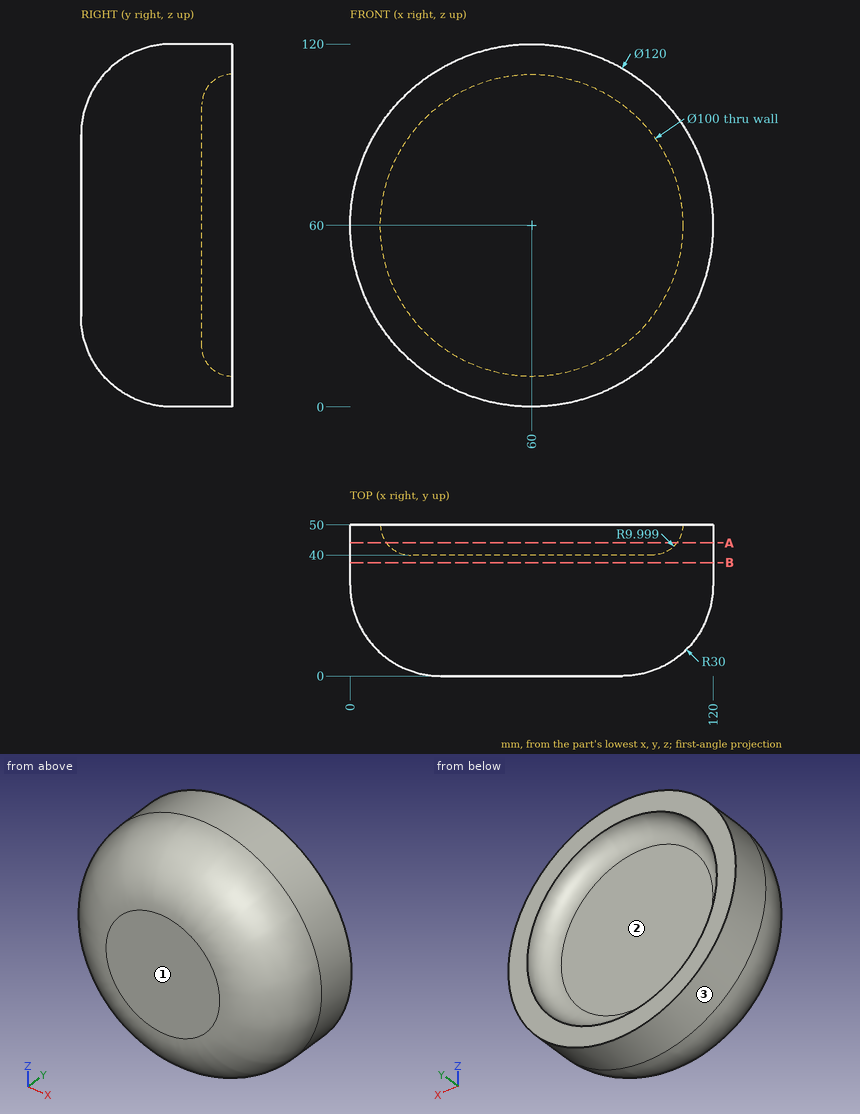
Source: three-view drawing plus pictorial views. Frame: mm from the lowest corner of the part. Give positions to 0.01 mm unless a question says otherwise; leave off trailing zeros. Loops run counter-clockwise (first coordinate to the right, second up) from the corner with the lowest first, then second, coordinate; pieces in that order, holes last. Notation, with made-up numbers: (-8, -21.5) -> (11, -21.5) arc R8 ccw to (11, -6.5) -> close; hole circle Ø4 at (87, -35.5). An arc over 180 degrees is marked (long way). Use a Markdown table: item, result. Add a question column.
(1) First-contact query: pin 1 Ø12 at (y, z) = (40.5, 88.5) entering from +X; pin 2 Ø1.5 at (x, z) = (94, 66) entering from -Y; pin 3 Ø6 at (y, z) = (39.5, 95) entering from -X (1 decimal). Flat tips, straight axial feed; report the tip coordinate or a pass-through.
(2) Section query B-B (y = 37.5). Output: boundary loops of the cut face in (x, z), then the cut area to 3 significant figures.
(3) Section query A-A (y = 44). Output: boundary loops of the cut face in (x, z).
(4) Ray query, line 1 (Y direction, x = 33.5, z = 49.5); line 2 (Z direction, x = 71.5, y = 43.5) (1 decimal); line 3 (Z direction, x = 107, y = 28). Return the intervals inside material, ascending.
(5) Pull-direction query (Z, two-part tool) for the marked faces 1, 2 and 3; classes: +Z half, -Z half, draft (parallel to the pull), parting line (faces both ways), or undercut.
Checked values:
| question | item | result |
|---|---|---|
| 1 | pin 1 | x = 115.62 |
| 1 | pin 2 | y = 0.24 |
| 1 | pin 3 | x = 9.2 |
| 2 | outline | circle Ø120 at (60, 60) |
| 2 | area | 11,300 mm^2 |
| 3 | outline | circle Ø120 at (60, 60); hole circle Ø96 at (60, 60) |
| 4 | line 1 | 0 to 40 |
| 4 | line 2 | 1.1 to 13.8, 106.2 to 118.9 |
| 4 | line 3 | 22.81 to 97.19 |
| 5 | face 1 | draft |
| 5 | face 2 | undercut |
| 5 | face 3 | parting line |
